Read the model definition and answer for the solid it produces. Units are mm, in the model's axes. Face numbers are marked on the shaded views. A direction names the side the tool comes from. Round coordinates to 2 decimals unless told otherwise and drop trailing zeros. Order: outer loops, then holes, each group sorted by start corner. A loop starts at its lowest first (then second) coordinate and runs counter-clockwise, first axis right, second up. Notation, with made-up numbers: (-29.5, 23.25) -> (-18.5, 23.25) arc R13 cw to (-18.5, 47.25) -> close; hole circle Ø9 at (20.5, -27). An arc over 180 degrees is marked (long way). Answer as a JSON object with one key per item and string values. Group by question number.
Item 1: Section C-C, the plane z = 5 is taken. Write down the section's boundary in (x, y).
Item 2: Consider probe 1 along Y at (x, z) = (0, 4); probe 2 along X at (y, z) = (1.95, 2.5). Determine where each line is inside the solid, lowest interval first. Write a range as from..to.
Item 3: Section D-D, the plane y = -1.7 is taken. Write down the section's boundary in (x, z).
Item 4: Section A-A, the plane x = 0 is taken. Write down the section's boundary in (y, z), plus the area to 3 significant figures.
Item 5: For the marked faces 1, 2 and 3, determine the directions among +Z, -Z, +X, -X, +Y, -Y from which every point of the face is accessible in a straight line to the end or side of a thin tool.
Item 6: Given P1, Ø1, axis at y = -1, z = 7, coming from the -X side; P2, Ø1, axis at x = 6, z = 7, coming from the +Y side; P3, Ø5, axis at x = 5, z = 3.5, coming from the +Y side; P4, Ø5, axis at x = 3, z = 7.5, coming from the +Y side, each flat-ended and moving along its own axis, determine where each tip first touches the part or whether it passes through.
Item 7: The mould has two halves that part along Z. Classify the marked faces 4, 5 and 6: pulls with the +Z half, pulls with the -Z half, needs draft (parallel to the pull), parting line crosses it, or undercut.
Item 8: Section B-B, the plane y = 0 is taken. Write down the section's boundary in (x, z).
from build123d import *

# Parameters (mm, degrees)
SKETCH1_R           = 3
SKETCH1_R_2         = 2.25
BOSS_EXTRUDE1_DEPTH = 10
CUT_EXTRUDE3_START  = -3
SKETCH2_W           = 1.120885769
SKETCH2_H           = 2.257305728
CUT_EXTRUDE3_DEPTH  = 4
SKETCH3_R           = 1
BOSS_EXTRUDE2_DEPTH = 5
BOSS_EXTRUDE3_START = 5
SKETCH4_R           = 1
BOSS_EXTRUDE3_DEPTH = 5


with BuildPart() as part:
    # Sketch1 → Boss-Extrude1 (new body)
    with BuildSketch(Plane.XY):
        Circle(SKETCH1_R)
        Circle(SKETCH1_R_2, mode=Mode.SUBTRACT)
    extrude(amount=BOSS_EXTRUDE1_DEPTH)

    # Sketch2 → Cut-Extrude3 (cut)
    with BuildSketch(Plane.XY.offset(10).offset(CUT_EXTRUDE3_START)):
        with Locations((-3.340036868, 0)):
            Rectangle(SKETCH2_W, SKETCH2_H)
        with Locations((3.340036868, 0)):
            Rectangle(SKETCH2_W, SKETCH2_H)
    extrude(amount=-CUT_EXTRUDE3_DEPTH, mode=Mode.SUBTRACT)

    # Sketch3 → Boss-Extrude2 (add)
    with BuildSketch(Plane.ZY.offset(2.779593983)):
        with Locations(Location((5, 0, 0), (0, 0, 90))):
            Circle(SKETCH3_R)
    extrude(amount=BOSS_EXTRUDE2_DEPTH)

    # Sketch4 → Boss-Extrude3 (add)
    with BuildSketch(Plane(origin=(2.779593983, 0, 0), x_dir=(0, 0, -1), z_dir=(1, 0, 0)).offset(BOSS_EXTRUDE3_START)):
        with Locations(Location((-5, 0, 0), (0, 0, 90))):
            Circle(SKETCH4_R)
    extrude(amount=-BOSS_EXTRUDE3_DEPTH)


solid = part.part
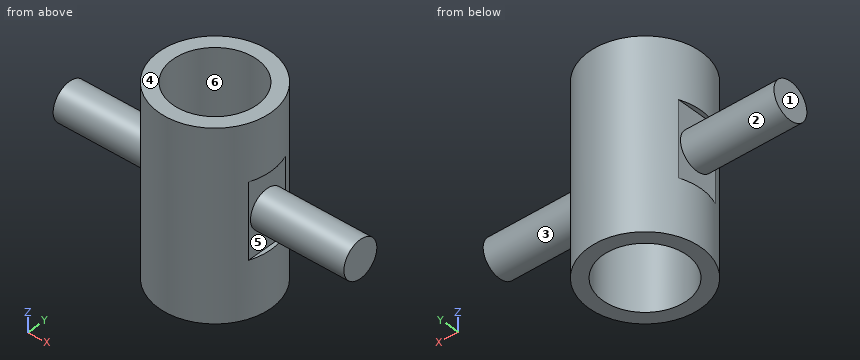
Values found:
{
 "1": {"outline": "(-7.78, -1) -> (-2.78, -1) -> (-2.78, -1.13) arc R3 ccw to (2.78, -1.13) -> (2.78, -1) -> (7.78, -1) -> (7.78, 1) -> (2.78, 1) -> (2.78, 1.13) arc R3 ccw to (-2.78, 1.13) -> (-2.78, 1) -> (-7.78, 1) -> close; hole circle Ø4.5 at (0, 0)"},
 "2": {"probe 1": "-3..-2.25, 2.25..3", "probe 2": "-2.28..-1.12, 1.12..2.28"},
 "3": {"outline": "(-2.47, 0) -> (-1.47, 0) -> (-1.47, 10) -> (-2.47, 10) -> close; (1.47, 0) -> (2.47, 0) -> (2.47, 10) -> (1.47, 10) -> close"},
 "4": {"outline": "(-3, 0) -> (-2.25, 0) -> (-2.25, 10) -> (-3, 10) -> close; (2.25, 0) -> (3, 0) -> (3, 10) -> (2.25, 10) -> close", "area": "15.0 mm2"},
 "5": {"face 1": "+Z, -Z, -X, +Y, -Y", "face 2": "-X", "face 3": "+X"},
 "6": {"P1": "x = -2.96", "P2": "through", "P3": "y = 1.66", "P4": "y = 2.96"},
 "7": {"face 4": "pulls with the +Z half", "face 5": "undercut", "face 6": "needs draft"},
 "8": {"outline": "(-7.78, 4) -> (-2.78, 4) -> (-2.78, 3) -> (-3, 3) -> (-3, 0) -> (-2.25, 0) -> (-2.25, 10) -> (-3, 10) -> (-3, 7) -> (-2.78, 7) -> (-2.78, 6) -> (-7.78, 6) -> close; (2.25, 0) -> (3, 0) -> (3, 3) -> (2.78, 3) -> (2.78, 4) -> (7.78, 4) -> (7.78, 6) -> (2.78, 6) -> (2.78, 7) -> (3, 7) -> (3, 10) -> (2.25, 10) -> close"}
}
